```python
from build123d import *

# Parameters (mm, degrees)
SCHIZZO1_W                   = 41
SCHIZZO1_H                   = 41
ESTRUSIONE_ESTRUSIONE1_DEPTH = 1.5
SCHIZZO5_W                   = 4.5
SCHIZZO5_H                   = 4.5
ESTRUSIONE_ESTRUSIONE2_DEPTH = 6.97
SCHIZZO6_W                   = 4.5
SCHIZZO6_H                   = 4.5
ESTRUSIONE_ESTRUSIONE3_DEPTH = 6.97
SCHIZZO7_W                   = 4.5
SCHIZZO7_H                   = 4.5
ESTRUSIONE_ESTRUSIONE4_DEPTH = 6.97
SCHIZZO8_W                   = 4.5
SCHIZZO8_H                   = 4.5
ESTRUSIONE_ESTRUSIONE5_DEPTH = 6.97
SCHIZZO9_W                   = 1
SCHIZZO9_H                   = 41
ESTRUSIONE_ESTRUSIONE6_DEPTH = 12
SCHIZZO10_W                  = 26
SCHIZZO10_H                  = 1
ESTRUSIONE_ESTRUSIONE7_DEPTH = 12
SCHIZZO11_R                  = 0.4
TAGLIO_ESTRUSIONE1_DEPTH     = 10
SCHIZZO12_R                  = 0.4
TAGLIO_ESTRUSIONE2_DEPTH     = 10


with BuildPart() as part:
    # Schizzo1 → Estrusione-Estrusione1 (new body)
    with BuildSketch(Plane.XY):
        with Locations((20.5, 20.5)):
            Rectangle(SCHIZZO1_W, SCHIZZO1_H)
    extrude(amount=ESTRUSIONE_ESTRUSIONE1_DEPTH)

    # Schizzo5 → Estrusione-Estrusione2 (add)
    with BuildSketch(Plane.XY.offset(1.5)):
        with Locations((2.25, 2.25)):
            Rectangle(SCHIZZO5_W, SCHIZZO5_H)
    extrude(amount=ESTRUSIONE_ESTRUSIONE2_DEPTH)

    # Schizzo6 → Estrusione-Estrusione3 (add)
    with BuildSketch(Plane.XY.offset(1.5)):
        with Locations((38.75, 2.25)):
            Rectangle(SCHIZZO6_W, SCHIZZO6_H)
    extrude(amount=ESTRUSIONE_ESTRUSIONE3_DEPTH)

    # Schizzo7 → Estrusione-Estrusione4 (add)
    with BuildSketch(Plane.XY.offset(1.5)):
        with Locations((2.25, 38.75)):
            Rectangle(SCHIZZO7_W, SCHIZZO7_H)
    extrude(amount=ESTRUSIONE_ESTRUSIONE4_DEPTH)

    # Schizzo8 → Estrusione-Estrusione5 (add)
    with BuildSketch(Plane.XY.offset(1.5)):
        with Locations((38.75, 38.75)):
            Rectangle(SCHIZZO8_W, SCHIZZO8_H)
    extrude(amount=ESTRUSIONE_ESTRUSIONE5_DEPTH)

    # Schizzo9 → Estrusione-Estrusione6 (add)
    with BuildSketch(Plane(origin=(0, 0, 0), x_dir=(-1, 0, 0), z_dir=(0, 0, -1))):
        with Locations((-40.5, 20.5)):
            Rectangle(SCHIZZO9_W, SCHIZZO9_H)
    extrude(amount=ESTRUSIONE_ESTRUSIONE6_DEPTH)

    # Schizzo10 → Estrusione-Estrusione7 (add)
    with BuildSketch(Plane(origin=(0, 0, 0), x_dir=(-1, 0, 0), z_dir=(0, 0, -1))):
        with Locations((-13, 40.5)):
            Rectangle(SCHIZZO10_W, SCHIZZO10_H)
    extrude(amount=ESTRUSIONE_ESTRUSIONE7_DEPTH)

    # Schizzo11 → Taglio-Estrusione1 (cut)
    with BuildSketch(Plane.XY.offset(8.47)):
        with Locations((38.781075858, 38.7)):
            Circle(SCHIZZO11_R)
    extrude(amount=-TAGLIO_ESTRUSIONE1_DEPTH, mode=Mode.SUBTRACT)

    # Schizzo12 → Taglio-Estrusione2 (cut)
    with BuildSketch(Plane.XY.offset(8.47)):
        with Locations((2.481075858, 2.5)):
            Circle(SCHIZZO12_R)
    extrude(amount=-TAGLIO_ESTRUSIONE2_DEPTH, mode=Mode.SUBTRACT)


solid = part.part
```
Input: part model. Units: mm. Frame: model coordinates. A direction names the side the tool comes from. Give positions to 0.01 mm unless a question says otherwise; leave off trailing zeros. Order: outer loops, then holes, each group sorted by start corner. A loop starts at its lowest first (then second) coordinate and runs counter-clockwise, first axis right, second up.
1. Set-up query: faces 1 (the face through (2, 4.5, 5)), 2 (the face through (4.5, 2, 5)), 3 (the face through (2, 39, 8.47)). Return all of +Z, -Z, +X, -X, +Y, -Y with unobstructed straight access to the full face (end or side cutting, diameter ignored); none if empty.
Computed:
face 1: +Z, +X, -X
face 2: +Z, +Y, -Y
face 3: +Z, +X, -X, +Y, -Y
2. Cut plane A-A (z = 4.25). Return loops of the section in (x, y), and give its area (3 significant figures).
Computed:
outline: (0, 0) - (4.5, 0) - (4.5, 4.5) - (0, 4.5) - close; (0, 36.5) - (4.5, 36.5) - (4.5, 41) - (0, 41) - close; (36.5, 0) - (41, 0) - (41, 4.5) - (36.5, 4.5) - close; (36.5, 36.5) - (41, 36.5) - (41, 41) - (36.5, 41) - close; hole circle Ø0.8 at (2.48, 2.5); hole circle Ø0.8 at (38.78, 38.7)
area: 80.0 mm2
3. Cut plane C-C (z = -0.75). Return loops of the section in (x, y).
Computed:
outline: (0, 40) - (26, 40) - (26, 41) - (0, 41) - close; (40, 0) - (41, 0) - (41, 41) - (40, 41) - close
4. Pin query (flat end, axial travel): pin 1 Ø8 at (x, y) = (22, 26.5) entering from -Z; pin 2 Ø9.5 at (x, z) = (7.5, -5.5) entering from -Y; pin 3 Ø3 at (y, z) = (14, -5) entering from -X. Return the tip coordinate at first contact, or that it passes through.
Computed:
pin 1: stops at z = 0
pin 2: stops at y = 40
pin 3: stops at x = 40
5. Cut plane B-B (x = 25). Return loops of the section in (y, z).
Computed:
outline: (0, 0) - (40, 0) - (40, -12) - (41, -12) - (41, 1.5) - (0, 1.5) - close
6. Line query: probe 1 along X at (y, z) = (38.7, 5); probe 2 along Y at (x, z) = (3.5, -9.75). Output: solid intervals per line, ascending.
Computed:
probe 1: x = 0 to 4.5, 36.5 to 38.38, 39.18 to 41
probe 2: y = 40 to 41
7. Draft query along X for faces 4 (the face through (40.5, 20.8, -12)), 5 (the face through (41, 20, -4)), 6 (the face through (36.5, 2, 5)). Return one class per face: released by +X, released by -X, zero draft, split by the parting line, or undercut.
Computed:
face 4: zero draft
face 5: released by +X
face 6: undercut
